```python
from build123d import *

# Parameters (mm, degrees)
SKETCH_1_W          = 10
SKETCH_1_H          = 10
SKETCH_1_R          = 3
EXTRUDE_1_DEPTH     = 2.5
SKETCH_3_W          = 10
SKETCH_3_H          = 10.5
EXTRUDE_2_DEPTH     = 2
SKETCH_3_3_R        = 0.6
CUT_EXTRUDE_1_DEPTH = 13.932517156
CUT_EXTRUDE_START   = -2
SKETCH_3_4_R        = 1
CUT_EXTRUDE_2_DEPTH = 1
FILLET_1_R          = 3
FILLET_2_R          = 3


with BuildPart() as part:
    # 草图1 → 凸台-拉伸1 (new body)
    with BuildSketch(Plane(origin=(0, 0, 0), x_dir=(1, 0, 0), z_dir=(0, 1, 0))):
        Rectangle(SKETCH_1_W, SKETCH_1_H)
        with Locations(Location((0, 0, 0), (0, 0, 270))):
            Circle(SKETCH_1_R, mode=Mode.SUBTRACT)
    extrude(amount=EXTRUDE_1_DEPTH)

    # 草图3 → 凸台-拉伸2 (add)
    with BuildSketch(Plane.ZY.offset(5)):
        with Locations((0, 1.25)):
            Rectangle(SKETCH_3_W, SKETCH_3_H)
    extrude(amount=-EXTRUDE_2_DEPTH)

    # 草图3<3> → 切除-拉伸1 (cut, through all)
    with BuildSketch(Plane.ZY.offset(5)):
        with Locations((-2, 4.25)):
            Circle(SKETCH_3_3_R)
        with Locations((2, 4.25)):
            Circle(SKETCH_3_3_R)
        with Locations((-2, -1.75)):
            Circle(SKETCH_3_3_R)
        with Locations((2, -1.75)):
            Circle(SKETCH_3_3_R)
    extrude(amount=-CUT_EXTRUDE_1_DEPTH, mode=Mode.SUBTRACT)

    # 草图3<4> → 切除-拉伸2 (cut)
    with BuildSketch(Plane.ZY.offset(5).offset(CUT_EXTRUDE_START)):
        with Locations(Location((-2, 4.25, 0), (0, 0, 180))):
            Circle(SKETCH_3_4_R)
        with Locations(Location((2, 4.25, 0), (0, 0, 180))):
            Circle(SKETCH_3_4_R)
        with Locations(Location((-2, -1.75, 0), (0, 0, 180))):
            Circle(SKETCH_3_4_R)
        with Locations(Location((2, -1.75, 0), (0, 0, 180))):
            Circle(SKETCH_3_4_R)
    extrude(amount=CUT_EXTRUDE_2_DEPTH, mode=Mode.SUBTRACT)

    # 圆角1
    fillet_1_edges = [part.edges().sort_by_distance(p)[0] for p in [
        (5, 1.25, 5),
        (5, 1.25, -5),
    ]]
    fillet(fillet_1_edges, radius=FILLET_1_R)

    # 圆角2
    fillet_2_edges = [part.edges().sort_by_distance(p)[0] for p in [
        (-4, 6.5, 5),
        (-4, 6.5, -5),
        (-4, -4, 5),
        (-4, -4, -5),
    ]]
    fillet(fillet_2_edges, radius=FILLET_2_R)


solid = part.part
```
The model under review builds one solid part; all positions refer to its coordinate system, in mm. A direction names the side the tool comes from. Coordinates: 2 decimals unless noted, no trailing zeros. Order: outer loops, then holes, each group sorted by start corner. A loop starts at its lowest first (then second) coordinate and runs counter-clockwise, first axis right, second up. Notation, with made-up numbers: (24, 44) -> (31, 44) arc R19 ccw to (31, 72) -> close; hole circle Ø2 at (62.25, 61.5). An arc over 180 degrees is marked (long way). Answer in a Markdown table with one row per item. Add a question column.
Item 1: Clearance check with flat-ended pins moving along their axes: pin 1 (2.5 mm diameter, centred on y = -1.75, z = -2, fed in from +X); pin 2 (1 mm diameter, centred on y = -1.5, z = -2, fed in from +X); pin 3 (1.5 mm diameter, centred on x = 4, y = 2.5, fed in from -Z). State where each tip first meets the part, or that it passes through.
Item 2: Mouldability with a two-part tool opening along Y and no side actions: class faces 1 (the cylindrical face through (-4.507, 3.664, 1.87)), 2 (the flat face through (-2, 1, -5)), 3 (the cylindrical face through (-3.99, 5.6, -4.14)), 4 (the flat face through (4, 0, 0)) as +Y half, -Y half, draft (parallel to the pull), parting line (faces both ways), or undercut.
Item 3: We need section D-D on y = 0.5. Write out the cut boundary in (x, z).
Item 4: We need section B-B on y = -2. Write out the cut boundary in (x, z).
Item 5: We need section A-A on x = -3.25. Write out the cut boundary in (y, z).
Item 6: Machinability: for faces 5 (the flat face through (-3, 5, 0)), 6 (the cylindrical face through (-3.5, -1.8, 3)), 7 (the flat face through (-3, -2, 0)), which of the approach directions +Z, -Z, +X, -X, +Y, -Y give a long, thin tool a straight path to every point of the face, cutting with its end or side? Answer none if there is none.
Item 7: To check wall thickness, follow probe 1 along Y at (x, z) = (-4.6, -2); probe 2 along Y at (x, z) = (-3.15, -2); probe 3 along Z at (x, y) = (-3.65, 4.25). State the ranges of each line that lie inside material, in increasing order.
Item 8: We need section C-C on z = 0.5. Write out the cut boundary in (x, y), plus the area to 3 significant figures.
Final values:
| question | item | result |
|---|---|---|
| 1 | pin 1 | stops at x = -3 |
| 1 | pin 2 | stops at x = -4 |
| 1 | pin 3 | stops at z = -4.73 |
| 2 | face 1 | undercut |
| 2 | face 2 | draft |
| 2 | face 3 | +Y half |
| 2 | face 4 | -Y half |
| 3 | outline | (-5, -5) -> (2, -5) arc R3 ccw to (5, -2) -> (5, 2) arc R3 ccw to (2, 5) -> (-5, 5) -> close; hole circle Ø6 at (0, 0) |
| 4 | outline | (-5, -4.83) -> (-3, -4.83) -> (-3, -2.97) -> (-4, -2.97) -> (-4, -2.55) -> (-5, -2.55) -> close; (-5, -1.45) -> (-4, -1.45) -> (-4, -1.03) -> (-3, -1.03) -> (-3, 1.03) -> (-4, 1.03) -> (-4, 1.45) -> (-5, 1.45) -> close; (-5, 2.55) -> (-4, 2.55) -> (-4, 2.97) -> (-3, 2.97) -> (-3, 4.83) -> (-5, 4.83) -> close |
| 5 | outline | (-4, -2) arc R3 ccw to (-1, -5) -> (3.5, -5) arc R3 ccw to (6.5, -2) -> (6.5, 2) arc R3 ccw to (3.5, 5) -> (-1, 5) arc R3 ccw to (-4, 2) -> close; hole circle Ø2 at (-1.75, -2); hole circle Ø2 at (-1.75, 2); hole circle Ø2 at (4.25, -2); hole circle Ø2 at (4.25, 2) |
| 6 | face 5 | +Z, -Z, +X, +Y |
| 6 | face 6 | +X |
| 6 | face 7 | +Z, -Z, +X, -Y |
| 7 | probe 1 | y = -4 to -2.35, -1.15 to 3.65, 4.85 to 6.5 |
| 7 | probe 2 | y = -4 to -2.75, -0.75 to 3.25, 5.25 to 6.5 |
| 7 | probe 3 | z = -4.9 to -3, -1 to 1, 3 to 4.9 |
| 8 | outline | (-5, -4) -> (-3, -4) -> (-3, 0) -> (-2.96, 0) -> (-2.96, 2.5) -> (-3, 2.5) -> (-3, 6.5) -> (-5, 6.5) -> close; (2.96, 0) -> (5, 0) -> (5, 2.5) -> (2.96, 2.5) -> close |
| 8 | area | 26.2 mm2 |
